Input: part model. Units: mm. Frame: model coordinates. Face numbers are marked on the shaded views. Round coordinates to 2 decimals unless told otherwise and drop trailing zeros. Order: outer loops, then holes, each group sorted by start corner. A loop starts at its lowest first (then second) coordinate and runs counter-clockwise, first axis right, second up.
Item 1: Cut plane A-A on z = -61. Give the number of separate pieces and of enclosed holes in the cut face, then the cut area to 3 significant figures.
Item 2: Line query: L1, parallel to Z at x = 0, y = -4.5; L2, parallel to X at y = -135, z = -75; L3, parallel to X at y = -48.5, z = -12.5. Output: solid intervals per line, ascending.
Item 3: First-contact query: pin 1 (2.5 mm diameter, centred on y = -6.5, z = -229.5, fed in from -X); pin 2 (3 mm diameter, centred on x = 182, y = -40, fed in from +Z); pin 3 (5 mm diameter, centred on y = -46.5, z = 19, fed in from -X). Flat tips, straight axial feed; report the tip coordinate or a pass-through.
Item 4: Cut plane B-B on y = -23. Output: boundary loops of the cut face in (x, z), then the cut area to 3 significant figures.
Item 5: Mould query, pull axis Z, two halves, no side actions, for the marked faces 1, 2 and 3. Classes: released by +Z, released by -Z, zero draft, split by the parting line, or undercut.
Item 6: Cut plane C-C on y = -93.5. Output: boundary loops of the cut face in (x, z).
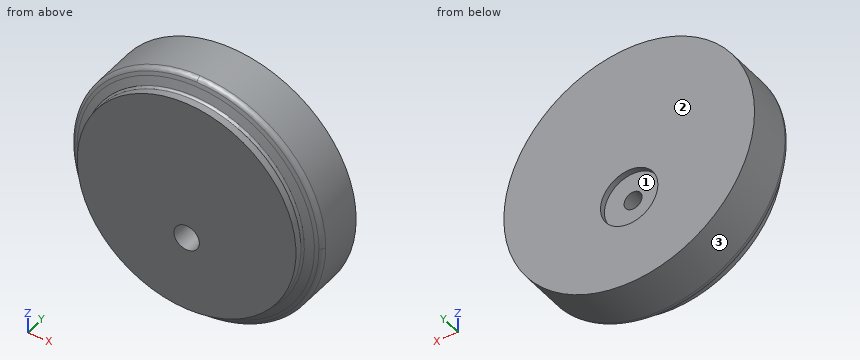
```python
from build123d import *

# Parameters (mm, degrees)
F0_R     = 284
F1_DEPTH = 147
F3_D     = 40
F4_R     = 28.815
F5_DEPTH = 200
F5_TAPER = 3.58
F7_R     = 65
F8_DEPTH = 13
F11_R    = 13


with BuildPart() as f1:
    # F0 (on Front) → F1 (new body)
    with BuildSketch(Plane.XZ):
        Circle(F0_R)
    extrude(amount=F1_DEPTH)

    # F3 (through all)
    with Locations(Plane.XZ.offset(147)):
        with Locations((0, -76)):
            Hole(F3_D / 2)

    # F4 (on face) → F5 (cut)
    with BuildSketch(Plane.XZ.offset(147)):
        with Locations((0, -76)):
            Circle(F4_R)
    extrude(amount=-F5_DEPTH, taper=F5_TAPER, mode=Mode.SUBTRACT)

    # F7 (on face) → F8 (cut)
    with BuildSketch(Plane(origin=(0, 0, 0), x_dir=(-1, 0, 0), z_dir=(0, 1, 0))):
        with Locations((0, -76.0070607066)):
            Circle(F7_R)
    extrude(amount=-F8_DEPTH, mode=Mode.SUBTRACT)

    # F9 (on Right) → F10 (revolve, cut)
    with BuildSketch(Plane.YZ):
        with BuildLine():
            Line((-116.54, 268.8), (-102.9912134112, 297.8554666042))
            Line((-102.9912134112, 297.8554666042), (-166.7411327362, 297.8554666042))
            Line((-166.7411327362, 297.8554666042), (-150.4560261965, 257.221698761))
            Line((-150.4560261965, 257.221698761), (-162.0599727805, 247.8))
            Line((-162.0599727805, 247.8), (-130.4097104904, 247.8))
            ThreePointArc((-130.4097104904, 247.8), (-126.970992997, 248.8022947468), (-124.6093406534, 251.4952431249))
            Line((-124.6093406534, 251.4952431249), (-116.54, 268.8))
        make_face()
    revolve(axis=Axis((0, -103.910677135, 0), (0, -1, 0)), mode=Mode.SUBTRACT)

    # F11
    f11_edges = [f1.edges().sort_by_distance(p)[0] for p in [
        (-200.818326, -109.452124, -200.818326),
        (200.818326, -109.452124, 200.818326),
    ]]
    fillet(f11_edges, radius=F11_R)

    # F14: sweep along a path in F12
    with BuildLine(Plane(origin=(0, 0, 0), x_dir=(-1, 0, 0), z_dir=(0, 1, 0))) as f14_path:
        ThreePointArc((0, -228.1088728905), (122.7460108736, -165.7605143402), (144.7944915292, -29.8643572934))
    # F13 (on Right) → F14 (sweep, cut)
    with BuildSketch(Plane.YZ):
        with BuildLine():
            Line((-4.6, -230.45), (-4.6, -225.55))
            Line((-4.6, -225.55), (-8.0746106855, -224.0030036525))
            ThreePointArc((-8.0746106855, -224.0030036525), (-8.835711228, -224.0629035643), (-9.2, -224.7338400186))
            Line((-9.2, -224.7338400186), (-9.2, -227.7760519524))
            Line((-9.2, -227.7760519524), (-9.2, -228.2239480476))
            Line((-9.2, -228.2239480476), (-9.2, -231.2661599814))
            ThreePointArc((-9.2, -231.2661599814), (-8.835711228, -231.9370964357), (-8.0746106855, -231.9969963475))
            Line((-8.0746106855, -231.9969963475), (-4.6, -230.45))
        make_face()
    sweep(path=f14_path.line, mode=Mode.SUBTRACT)


solid = f1.part
```
From the geometry:
1. separate pieces: 2
1. enclosed holes: 1
1. area: 72,500 mm2
2. L1: z = -284 to -141.01, -11.01 to 284
2. L2: x = -236.18 to -28.05, 28.05 to 236.18
2. L3: x = -283.72 to 283.72
3. pin 1: stops at x = -168.99
3. pin 2: stops at z = 219.26
3. pin 3: stops at x = -283.52
4. outline: circle Ø568 at (0, 0); hole circle Ø42.11 at (0, -76)
4. area: 252,000 mm2
5. face 1: undercut
5. face 2: zero draft
5. face 3: split by the parting line
6. outline: circle Ø568 at (0, 0); hole circle Ø50.94 at (0, -76)
